The listing builds one solid part. Answer for the finished solid, in the listing's coordinates (mm). Face numbers are marked on the shaded views. Round coordinates to 2 decimals unless told otherwise and drop trailing zeros. Order: outer loops, then holes, each group sorted by start corner. A loop starts at its lowest first (then second) coordinate and runs counter-clockwise, first axis right, second up. Notation, with made-up numbers: M 6.5,-32.5 L 25.5,-32.5 A23 cw 25.5,-13.5 Z; hole C 78.5,-37 d1. An arc over 180 degrees is marked long. Write item = value, one per line. Start each with the question number.
(1) Straight lines are drawn through the part: probe 1 along X at (y, z) = (879.5, 1304.2); probe 2 along Y at (x, z) = (673, 1302.7); probe 3 along Y at (x, z) = (680, 1303.2). For each, find the intervals that lie inside material, in ascending order. Write a range as from..to.
(2) A cutting plane is placed at A-A, the plane z = 1303. Determine the outline of the cut face in (x, y).
(3) Each of these flat-tipped pins is pushed along its axis until it touches: pin 1 (1 mm diameter, centred on x = 689.5, z = 1303.5, fed in from -Y); pin 2 (2.5 mm diameter, centred on x = 699.98, y = 875.2, fed in from -Z). Where does it stop, or does it pass through?
(4) For a pull along X with two mould halves and no side action, classify the marked faces 1 and 2 as released by +X, released by -X, zero draft, split by the parting line, or undercut.
from build123d import *

# Parameters (mm, degrees)
SKETCH1_R           = 25
SKETCH1_R_2         = 6
SKETCH1_R_3         = 1
BOSS_EXTRUDE1_DEPTH = 3
FILLET1_R           = 1


with BuildPart() as part:
    # Sketch1 → Boss-Extrude1 (new body)
    with BuildSketch(Plane.XY.offset(1301.677843453)):
        with Locations((678.383867879, 875.198049015)):
            Circle(SKETCH1_R)
        with Locations((678.383867879, 875.198049015)):
            Circle(SKETCH1_R_2, mode=Mode.SUBTRACT)
        with Locations((678.383867879, 896.799115491)):
            Circle(SKETCH1_R_3, mode=Mode.SUBTRACT)
        with Locations((678.383867879, 853.59698254)):
            Circle(SKETCH1_R_3, mode=Mode.SUBTRACT)
        with Locations((699.984934354, 875.198049015)):
            Circle(SKETCH1_R_3, mode=Mode.SUBTRACT)
        with Locations((656.782801404, 875.198049015)):
            Circle(SKETCH1_R_3, mode=Mode.SUBTRACT)
    extrude(amount=BOSS_EXTRUDE1_DEPTH)

    # Fillet1
    fillet1_edges = [part.edges().sort_by_distance(p)[0] for p in [
        (653.383867879, 875.198049015, 1304.677843453),
    ]]
    fillet(fillet1_edges, radius=FILLET1_R)


solid = part.part
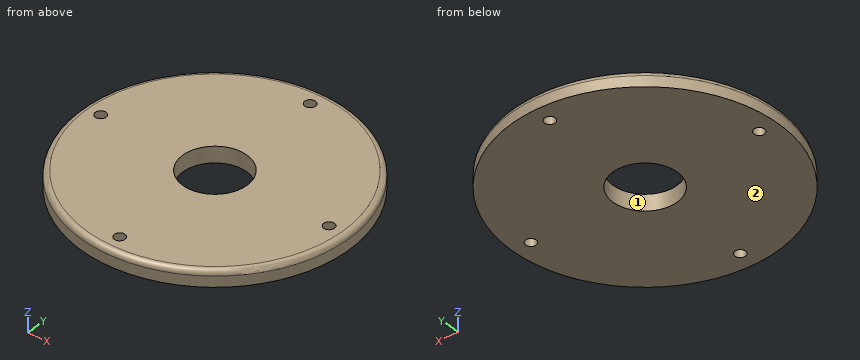
Reported:
q1.probe_1 = 653.91..674.2, 682.57..702.86
q1.probe_2 = 850.78..872.55, 877.85..899.61
q1.probe_3 = 850.25..869.42, 880.98..900.15
q2.outline = C 678.38,875.2 d50; hole C 656.78,875.2 d2; hole C 678.38,875.2 d12; hole C 678.38,853.6 d2; hole C 678.38,896.8 d2; hole C 699.98,875.2 d2
q3.pin_1 = 852.56
q3.pin_2 = 1301.68
q4.face_1 = undercut
q4.face_2 = zero draft
